Here's how the part is built. I have some questions about the finished solid (model axes, mm). A direction names the side the tool comes from. Coordinates: 2 decimals unless noted, no trailing zeros. Loops run counter-clockwise (first coordinate to the right, second up) from the corner with the lowest first, then second, coordinate; pieces in that order, holes last. Notation, with made-up numbers: M 68.25,43.25 L 86.25,43.25 A19 cw 86.25,59.25 Z; hole C -38.5,53.25 d9. An arc over 180 degrees is marked long. Use one line per item in the form item = value. Start each with the question number.
(1) Imagine slicing it at B-B, the plane z = 8.25. Please give me the cut outline in (x, y), and give its area (3 significant figures).
(2) Imagine slicing it at C-C, the plane y = 116. Please give me the cut outline in (x, z).
(3) Imagine slicing it at A-A, the plane y = 190.5. Please give me the cut outline in (x, z), and give its area (3 significant figures).
(4) Thinking about a two-plate mould opening in X: for faces 1 (the cylindrical face through (-74.03, 246.04, 4.93)), 2 (the flat face through (-37, 193, 10)), 3 (the cylindrical face through (155.048, 54.213, 4.93)), which applies, +X half, -X half, draft (parallel to the pull), parting line (faces both ways), or undercut?
(5) Imagine slicing it at D-D, the plane x = 0. Please give me the cut outline in (y, z).
(6) Please list where these lines run through material, in increasing order: L1, parallel to X at y = 57.5, z = 7; L2, parallel to X at y = 41, z = 3; L3, parallel to Y at x = 33.5, z = 2.5.
(7) On a 3-axis mill with a long thin cutter (end or side, diameter ignored), from which of +Z, -Z, +X, -X, +Y, -Y can I reach the whole of each face in a straight line? I mean faces 4 (the flat face through (-37, 193, 0)), 5 (the flat face through (90, 56, 5)). Say none if no direction works.
(8) Will these pins go through, and if not, where does the flat tip stop? P1, Ø6, axis at x = -98, y = 69, coming from the -Z side; P2, Ø5, axis at y = 36.5, z = 6, coming from the -X side; P3, Ø3, axis at x = -28.5, z = 7.5, coming from the +Y side; P4, Ø6, axis at x = 69.5, z = 3.5, coming from the -Y side.
```python
from build123d import *

# Parameters (mm, degrees)
F2_DEPTH = 10


with BuildPart() as f2:
    # F1 (on Top) → F2 (new body)
    with BuildSketch(Plane.XY):
        with BuildLine():
            ThreePointArc((-105, 110), (0, 215), (105, 110))
            Line((105, 110), (105, 0))
            Line((105, 0), (145, 0))
            Line((145, 0), (145, 110))
            ThreePointArc((145, 110), (142.2138656585, 138.2880966923), (133.9625322141, 165.4890976929))
            ThreePointArc((133.9625322141, 165.4890976929), (118.7770464219, 193.1685832709), (97.9605801043, 216.9052138375))
            ThreePointArc((97.9605801043, 216.9052138375), (69.7433714933, 237.1253795776), (37.5287615399, 250.0592448119))
            ThreePointArc((37.5287615399, 250.0592448119), (0, 255), (-37.5287615399, 250.0592448119))
            ThreePointArc((-37.5287615399, 250.0592448119), (-69.7433714933, 237.1253795776), (-97.9605801043, 216.9052138375))
            ThreePointArc((-97.9605801043, 216.9052138375), (-118.7770464219, 193.1685832709), (-133.9625322141, 165.4890976929))
            ThreePointArc((-133.9625322141, 165.4890976929), (-142.2138656585, 138.2880966923), (-145, 110))
            Line((-145, 110), (-145, 0))
            Line((-145, 0), (-105, 0))
            Line((-105, 0), (-105, 110))
        make_face()
        with BuildLine():
            ThreePointArc((-145, 110), (-155.0496837882, 55), (-145, 0))
            Line((-145, 0), (-145, 110))
        make_face()
        with BuildLine():
            ThreePointArc((-133.9625322141, 165.4890976929), (-151.8883856552, 140.2124783682), (-145, 110))
            ThreePointArc((-145, 110), (-142.2138656585, 138.2880966923), (-133.9625322141, 165.4890976929))
        make_face()
        with BuildLine():
            ThreePointArc((-97.9605801043, 216.9052138375), (-126.948851738, 198.890542954), (-133.9625322141, 165.4890976929))
            ThreePointArc((-133.9625322141, 165.4890976929), (-118.7770464219, 193.1685832709), (-97.9605801043, 216.9052138375))
        make_face()
        with BuildLine():
            ThreePointArc((-37.5287615399, 250.0592448119), (-74.4950323823, 245.7865136926), (-97.9605801043, 216.9052138375))
            ThreePointArc((-97.9605801043, 216.9052138375), (-69.7433714933, 237.1253795776), (-37.5287615399, 250.0592448119))
        make_face()
        with BuildLine():
            ThreePointArc((-37.5287615399, 250.0592448119), (0, 255), (37.5287615399, 250.0592448119))
            ThreePointArc((37.5287615399, 250.0592448119), (0, 264.8969025948), (-37.5287615399, 250.0592448119))
        make_face()
        with BuildLine():
            ThreePointArc((37.5287615399, 250.0592448119), (69.7433714933, 237.1253795776), (97.9605801043, 216.9052138375))
            ThreePointArc((97.9605801043, 216.9052138375), (74.4950323823, 245.7865136926), (37.5287615399, 250.0592448119))
        make_face()
        with BuildLine():
            ThreePointArc((97.9605801043, 216.9052138375), (118.7770464219, 193.1685832709), (133.9625322141, 165.4890976929))
            ThreePointArc((133.9625322141, 165.4890976929), (126.948851738, 198.890542954), (97.9605801043, 216.9052138375))
        make_face()
        with BuildLine():
            ThreePointArc((133.9625322141, 165.4890976929), (142.2138656585, 138.2880966923), (145, 110))
            ThreePointArc((145, 110), (151.8883856552, 140.2124783682), (133.9625322141, 165.4890976929))
        make_face()
        with BuildLine():
            Line((145, 110), (145, 0))
            ThreePointArc((145, 0), (155.0496837882, 55), (145, 110))
        make_face()
        with BuildLine():
            Line((105, 0), (105, 110))
            ThreePointArc((105, 110), (0, 215), (-105, 110))
            Line((-105, 110), (-105, 0))
            Line((-105, 0), (-90, 0))
            Line((-90, 0), (-90, 110))
            ThreePointArc((-90, 110), (0, 200), (90, 110))
            Line((90, 110), (90, 2.92e-08))
            Line((90, 0), (105, 0))
        make_face()
    extrude(amount=F2_DEPTH)


solid = f2.part
```
Answer:
q1.outline = M -145,0 L -90,0 L -90,110 A90 cw 90,110 L 90,0 L 145,0 A155.53 ccw 145,110 A37.95 ccw 133.96,165.49 A43.42 ccw 97.96,216.91 A49.33 ccw 37.53,250.06 A54.88 ccw -37.53,250.06 A49.33 ccw -97.96,216.91 A43.42 ccw -133.96,165.49 A37.95 ccw -145,110 A155.53 ccw Z
q1.area = 37,000 mm²
q2.outline = M -148.69,0 L -89.8,0 L -89.8,10 L -148.69,10 Z; M 89.8,0 L 148.69,0 L 148.69,10 L 89.8,10 Z
q3.outline = M -131.54,0 L -40.25,0 L -40.25,10 L -131.54,10 Z; M 40.25,0 L 131.54,0 L 131.54,10 L 40.25,10 Z
q3.area = 1,830 mm²
q4.face_1 = undercut
q4.face_2 = draft
q4.face_3 = +X half
q5.outline = M 200,0 L 264.9,0 L 264.9,10 L 200,10 Z
q6.L1 = -155.03 to -90, 90 to 155.03
q6.L2 = -154.42 to -90, 90 to 154.42
q6.L3 = 193.53 to 253.49
q7.face_4 = -Z, +X, -X, +Y, -Y
q7.face_5 = +Z, -Z, -Y
q8.P1 = 0
q8.P2 = -154.22
q8.P3 = 257.8
q8.P4 = 163.33
